Print and shaded views of the part. All mm, measured from the part's lowest x, y and z. A direction names the side the tool comes from. Coordinates: 2 decimals unless noted, no trailing zeros. Loops run counter-clockwise (first coordinate to the right, second up) from the corner with the lowest first, then second, coordinate; pieces in that order, holes last. Notation, with made-up numbers: (54, -24) -> (101, -24) arc R36 ccw to (101, 15) -> close; hole circle Ø10 at (27, -21). An arc over 180 degrees is marked (long way). One line per item, written item: value. Start each with the question number.
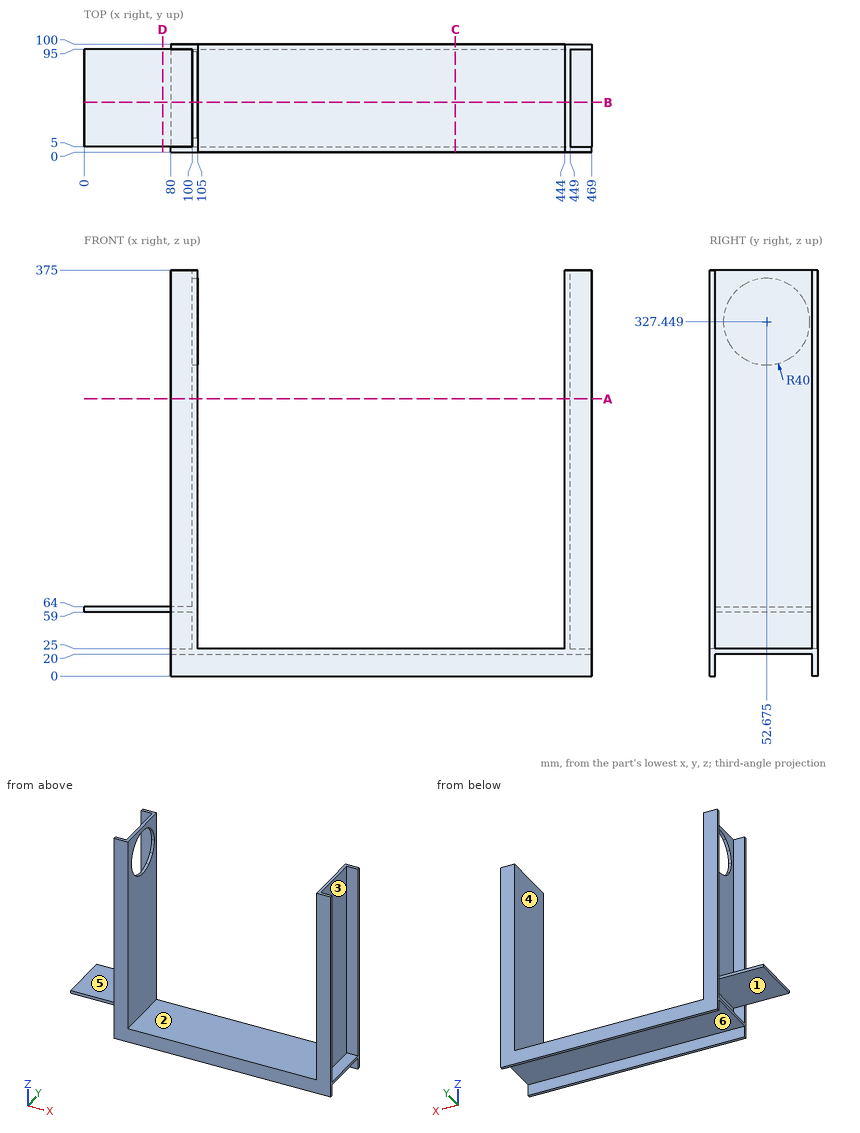
1) Tool access for the marked faces 4, 5 and 6: list every direction of +Z, -Z, +X, -X, +Y, -Y with a clear straight run to the whole face (end or side of a thin tool).
2) Pull direction X, two halves, no side cores. Call the marked faces 1, 2 and 3: +X half, -X half, draft (parallel to the pull), parting line (faces both ways), or undercut.
3) Probe line 1 (X direction, y = 89.5, z = 69); line 2 (X direction, y = 24.5, z = 60.5); line 3 (Z direction, x = 109, y = 44). List the from-to ranges inside material, lowest first. Write a range as from..to.
4) Slice it at C-C (x = 343). Give the cut face in (y, z), then the cut area to 3 significant figures.
5) Pin check, flat tips, straight feed: pin 1 Ø12 at (x, y) = (405.5, 16.5) entering from +Z; pin 2 Ø5 at (y, z) = (43, 131.5) entering from -X; pin 3 Ø4 at (x, y) = (400.5, 43.5) entering from -Z. Stop position of each tip, or through.
6) Slice it at D-D (x = 72.5). Give the cut face in (y, z), then the cut area to 3 significant figures.
7) Slice it at B-B (y = 46). Give the cut face in (x, z), then the cut area to 3 significant figures.
8) Slice it at A-A (z = 256). Give the cut face in (x, y), then the cut area to 3 significant figures.
Check sheet entries:
1. face 4: +Z, +Y, -Y
1. face 5: +Z, -X
1. face 6: -Z, +X, -X
2. face 1: draft
2. face 2: undercut
2. face 3: +X half
3. line 1: x = 100..105, 444..449
3. line 2: x = 0..105, 444..449
3. line 3: z = 20..25
4. outline: (0, 0) -> (5, 0) -> (5, 20) -> (95, 20) -> (95, 0) -> (100, 0) -> (100, 25) -> (0, 25) -> close
4. area: 700 mm^2
5. pin 1: stops at z = 25
5. pin 2: stops at x = 100
5. pin 3: stops at z = 20
6. outline: (5, 59) -> (95, 59) -> (95, 64) -> (5, 64) -> close
6. area: 450 mm^2
7. outline: (0, 59) -> (100, 59) -> (100, 25) -> (80, 25) -> (80, 20) -> (469, 20) -> (469, 25) -> (449, 25) -> (449, 375) -> (444, 375) -> (444, 25) -> (105, 25) -> (105, 288.01) -> (100, 288.01) -> (100, 64) -> (0, 64) -> close; (100, 366.89) -> (105, 366.89) -> (105, 375) -> (100, 375) -> close
7. area: 5,550 mm^2
8. outline: (80, 0) -> (105, 0) -> (105, 100) -> (80, 100) -> (80, 95) -> (100, 95) -> (100, 5) -> (80, 5) -> close; (444, 0) -> (469, 0) -> (469, 5) -> (449, 5) -> (449, 95) -> (469, 95) -> (469, 100) -> (444, 100) -> close
8. area: 1,400 mm^2
